Geometry check sheet. Reference: the model listing, model coordinates, mm. A direction names the side the tool comes from. Round coordinates to 2 decimals unless told otherwise and drop trailing zeros. Write each loop counter-clockwise with the first axis right and the second up, starting at its lowest first coordinate (ties: lowest second). Pieces come first, ordered by that corner, then holes. Notation, with made-up numbers: (-10.5, 19.25) - (30.5, 19.25) arc R33 ccw to (30.5, 48.25) - close; hole circle Ø4 at (72, 62.5). An arc over 180 degrees is marked (long way). Return JSON: item names as keys, results as strings.
Autodesk Inventor part; units mm, degrees
ref_plane "YZ Plane" through (0, 0, 0) normal (1, 0, 0) x (0, 1, 0)
ref_plane "XZ Plane" through (0, 0, 0) normal (0, 1, 0) x (-1, 0, 0)
ref_plane "XY Plane" through (0, 0, 0) normal (0, 0, 1) x (1, 0, 0)
sketch "Sketch1" plane through (0, 0, 0) normal (0, 0, 1) x (1, 0, 0)
  line L0 (-55, 0) -> (55, 0)
  line L1 (55, 0) -> (55, -130)
  line L2 (55, -130) -> (-55, -130)
  line L3 (-55, -130) -> (-55, 0)
  line L4 (0, 0) -> (0, -130)
  line L5 (-55, -65) -> (55, -65)
  circle A0 centre (40, -15) radius 5.35
  line L6 (55, -65) -> (-55, -65)
  circle A1 centre (-40, -15) radius 5.35
  circle A2 centre (40, -115) radius 5.35
  circle A3 centre (-40, -115) radius 5.35
  dimension "d0" = 110
  dimension "d1" = 130
  dimension "d2" = 10.7
  dimension "d3" = 40
  dimension "d4" = 50
extrude "Plate1" add sketch "Sketch1" along normal blind 3
sketch "Sketch2" plane through (0, 0, 3) normal (0, 0, 1) x (1, 0, 0)
  line L0 (13.5, -25) -> (16.5, -25)
  line L1 (16.5, -25) -> (16.5, -55)
  line L2 (16.5, -55) -> (13.5, -55)
  line L3 (13.5, -55) -> (13.5, -25)
  line L4 (0, 0) -> (0, -130)
  line L5 (-55, -130) -> (55, -130)
  line L6 (-55, 0) -> (55, 0)
  line L7 (-55, 0) -> (-55, -130)
  line L8 (-55, -65) -> (55, -65)
  line L9 (55, -130) -> (55, 0)
  line L10 (13.5, -105) -> (16.5, -105)
  line L11 (16.5, -105) -> (16.5, -75)
  line L12 (16.5, -75) -> (13.5, -75)
  line L13 (13.5, -75) -> (13.5, -105)
  line L14 (-13.5, -25) -> (-16.5, -25)
  line L15 (-16.5, -25) -> (-16.5, -55)
  line L16 (-16.5, -55) -> (-13.5, -55)
  line L17 (-13.5, -55) -> (-13.5, -25)
  line L18 (-13.5, -75) -> (-13.5, -105)
  line L19 (-16.5, -105) -> (-16.5, -75)
  line L20 (-13.5, -105) -> (-16.5, -105)
  line L21 (-16.5, -75) -> (-13.5, -75)
  line L22 (-15, -107) -> (15, -107)
  line L23 (15, -107) -> (15, -110)
  line L24 (15, -110) -> (-15, -110)
  line L25 (-15, -110) -> (-15, -107)
  point P0 (13.5, -40)
  point P1 (15, -25)
  point P2 (-15, -108.5)
  dimension "d6" = 3
  dimension "d7" = 30
  dimension "d8" = 13.5
  dimension "d9" = 25
  dimension "d10" = 30
  dimension "d11" = 3
  dimension "d12" = 15
  dimension "d13" = 20
extrude "Cut1" cut sketch "Sketch2" against normal blind 3 contours L0 L1 L2 L3 | L22 L23 L24 L4 | L4 L24 L25 L22 | L13 L12 L11 L10 | L17 L16 L15 L14 | L18 L20 L19 L21
chamfer "Corner Chamfer1" distance 6 angle 45 4 edges at (55, 0, 1.5) (-55, 0, 1.5) (-55, -130, 1.5) (55, -130, 1.5)
equation "\"d6\" = plate_thickness"
equation "\"d11\" = plate_thickness"
equation "\"d14\" = Thickness"
equation "\"d5\" = Thickness"
equation "\"Thickness\" = plate_thickness"
equation "\"BendRadius\" = Thickness"
equation "\"BendReliefWidth\" = Thickness"
equation "\"BendReliefDepth\" = 0.5 * Thickness"
equation "\"CornerReliefSize\" = 4 * Thickness"
equation "\"MinimumRemnant\" = 2 * Thickness"
equation "\"TransitionRadius\" = BendRadius"
equation "\"JacobiRadiusSize\" = BendRadius"
equation "\"GapSize\" = Thickness"
equation "\"A_width\" = 46"
equation "\"A_joint_diameter\" = 16"
equation "\"A_joint_tolerance\" = 3"
equation "\"l___________\" = 0"
equation "\"l__________\" = 0"
equation "\"l_________\" = 0"
equation "\"rivet_diameter\" = 3.35"
equation "\"plate_thickness\" = 3"
equation "\"l________\" = 0"
equation "\"L_Piston_Bottom\" = 21"
equation "\"L_Piston_Top\" = 25"
equation "\"A_B_spacing\" = 2"
equation "\"thin_plate\" = 1.5"
properties part number "Piston_FloorHinge_BasePlate" material "Stainless Steel"
(1) Access from +Z, -Z, +X, -X, +Y, -Y to the whole of each face (thin tool, end or side, straight path). Record for faces 1 (the face through (-1, -64, 3)), 2 (the face through (15, -105, 2)).
Response values:
{"face 1": "+Z, +X, -X, +Y, -Y", "face 2": "+Z, -Z"}
(2) Section check A-A, the plane y = -15. Enter the section's corners in (x, z), plus the area to 3 significant figures.
Response values:
{"outline": "(-55, 0) - (-45.35, 0) - (-45.35, 3) - (-55, 3) - close; (-34.65, 0) - (34.65, 0) - (34.65, 3) - (-34.65, 3) - close; (45.35, 0) - (55, 0) - (55, 3) - (45.35, 3) - close", "area": "266 mm^2"}
(3) Material ranges on line 1 along Y through (x, z) = (-40, 1.2); line 2 along X through (y, z) = (-97, 2.7); line 3 along Y through (x, z) = (-12, 1.75), recorded low to high. Write a range as [from, to].
Response values:
{"line 1": "y = [-130, -120.35], [-109.65, -20.35], [-9.65, 0]", "line 2": "x = [-55, -16.5], [-13.5, 13.5], [16.5, 55]", "line 3": "y = [-130, -110], [-107, 0]"}
(4) Section check B-B, the plane x = 40. Enter the section's corners in (y, z).
Response values:
{"outline": "(-130, 0) - (-120.35, 0) - (-120.35, 3) - (-130, 3) - close; (-109.65, 0) - (-20.35, 0) - (-20.35, 3) - (-109.65, 3) - close; (-9.65, 0) - (0, 0) - (0, 3) - (-9.65, 3) - close"}
(5) Release check for a two-part mould opening along Y. For faces 3 (the face through (-55, -66, 1)), 4 (the face through (-15, -75, 2)), 5 (the face through (1, -130, 1)), 6 (the face through (-15, -25, 2)) record: pulls with the +Y half, pulls with the -Y half, needs draft (parallel to the pull), parting line crosses it, or undercut.
Response values:
{"face 3": "needs draft", "face 4": "undercut", "face 5": "pulls with the -Y half", "face 6": "undercut"}
(6) Section check C-C, the plane z = 2.1. Give the number of separate pieces and of enclosed holes in the cut face, plus the area to 3 significant figures.
Response values:
{"separate pieces": "1", "enclosed holes": "9", "area": "13,400 mm^2"}
